Check sheet for the modelled part. Datum: model origin and axes. Units: mm. A direction names the side the tool comes from. Give positions to 0.01 mm unless a question says otherwise; leave off trailing zeros. Order: outer loops, then holes, each group sorted by start corner. A loop starts at its lowest first (then second) coordinate and runs counter-clockwise, first axis right, second up.
Item 1: Access from +Z, -Z, +X, -X, +Y, -Y to the whole of each face (thin tool, end or side, straight path). Record for faces 1 (the flat face through (143, 116, 0)), 2 (the flat face through (143, 117, -15)).
Item 2: Sectioned sample at C-C on y = 144. Record the boundary of the cut face in (x, z).
Item 3: Release check for a two-part mould opening along X. For faces 3 (the flat face through (275, 114, 39)), 4 (the flat face through (143, 15, 39)), 5 (the flat face through (0, 113, 33)), 6 (the flat face through (143, 230, 33)) record: released by +X, released by -X, zero draft, split by the parting line, or undercut.
Item 4: Sectioned sample at A-A on x = 174.5. Record the boundary of the cut face in (y, z), and give its area (3 significant figures).
Item 5: Material ranges on line 1 along Y through (x, z) = (257.5, 5.5); line 2 along X through (y, z) = (39, 32); line 3 along Z through (x, y) = (99, 93), recorded low to high.
Item 6: Sectioned sample at B-B on z = 57. Record the boundary of the cut face in (x, y), and give its area (3 significant figures).
Item 7: Gauge pin test, flat end, axial feed: P1, Ø4, axis at x = 166, y = 43, coming from the +Z side. Record the tip position at first contact, or that the pin passes through.
from build123d import *

# Parameters (mm, degrees)
SKETCH_1_W      = 290
SKETCH_1_H      = 230
SKETCH_1_W_2    = 260
SKETCH_1_H_2    = 200
EXTRUDE_1_DEPTH = 80
SKETCH_1_2_W    = 290
SKETCH_1_2_H    = 230
SKETCH_1_2_W_2  = 260
SKETCH_1_2_H_2  = 200
EXTRUDE_2_DEPTH = 15


with BuildPart() as part:
    # Sketch 1 → Extrude 1 (new body)
    with BuildSketch(Plane.XY):
        with Locations((145, 115)):
            Rectangle(SKETCH_1_W, SKETCH_1_H)
        with Locations((145, 115)):
            Rectangle(SKETCH_1_W_2, SKETCH_1_H_2, mode=Mode.SUBTRACT)
    extrude(amount=EXTRUDE_1_DEPTH)

    # Sketch 1_2 → Extrude 2 (add)
    # profile 1 of 2: a face of its own
    with BuildSketch(Plane.XY):
        with Locations((145, 115)):
            Rectangle(SKETCH_1_2_W, SKETCH_1_2_H)
        with Locations((145, 115)):
            Rectangle(SKETCH_1_2_W_2, SKETCH_1_2_H_2, mode=Mode.SUBTRACT)
    # profile 2 of 2: a face of its own
    with BuildSketch(Plane.XY):
        with Locations((145, 115)):
            Rectangle(SKETCH_1_2_W_2, SKETCH_1_2_H_2)
    extrude(amount=-EXTRUDE_2_DEPTH)


solid = part.part
Report:
1. face 1: +Z
1. face 2: -Z, +X, -X, +Y, -Y
2. outline: (0, -15) - (290, -15) - (290, 80) - (275, 80) - (275, 0) - (15, 0) - (15, 80) - (0, 80) - close
3. face 3: undercut
3. face 4: undercut
3. face 5: released by -X
3. face 6: zero draft
4. outline: (0, -15) - (230, -15) - (230, 80) - (215, 80) - (215, 0) - (15, 0) - (15, 80) - (0, 80) - close
4. area: 5,850 mm2
5. line 1: y = 0 to 15, 215 to 230
5. line 2: x = 0 to 15, 275 to 290
5. line 3: z = -15 to 0
6. outline: (0, 0) - (290, 0) - (290, 230) - (0, 230) - close; hole (15, 15) - (275, 15) - (275, 215) - (15, 215) - close
6. area: 14,700 mm2
7. P1: stops at z = 0
